from build123d import *

# Parameters (mm, degrees)
PAD_DEPTH       = 12
POCKET_DEPTH    = 10.1
POCKET001_DEPTH = 10.1
SKETCH003_W     = 15.841853
SKETCH003_H     = 14.91592
POCKET002_DEPTH = 4
SKETCH004_R     = 2
PAD001_DEPTH    = 2
CHAMFER_SIZE    = 0.5
CHAMFER001_SIZE = 1


with BuildPart() as part:
    # Sketch → Pad (new body)
    with BuildSketch(Plane.XY):
        Polygon((0, 7), (10, 7), (10, 0), (0, -10), (-7, -10), (-7, 0), (-4, 0), (0, 4), align=None)
    extrude(amount=PAD_DEPTH)

    # Sketch001 (on Face4 of Pad) → Pocket (cut)
    with BuildSketch(Plane.XZ.offset(10)):
        with BuildLine():
            Line((-4.5, 10), (-4.5, 13.32))
            Line((-4.5, 13.32), (-4, 13.32))
            Line((-4, 13.32), (-4, 4))
            ThreePointArc((-5, 4), (-4.5, 3.5), (-4, 4))
            Line((-5, 4), (-5, 9.5))
            Line((-5, 9.5), (-4.5, 10))
        make_face()
    extrude(amount=-POCKET_DEPTH, mode=Mode.SUBTRACT)

    # Sketch002 (on Face3 of Pocket) → Pocket001 (cut)
    with BuildSketch(Plane.YZ.offset(10)):
        with BuildLine():
            Line((4.5, 12.95), (4.5, 10))
            Line((4.5, 10), (5, 9.5))
            Line((5, 9.5), (5, 4))
            ThreePointArc((4, 4), (4.5, 3.5), (5, 4))
            Line((4, 4), (4, 12.95))
            Line((4, 12.95), (4.5, 12.95))
        make_face()
    extrude(amount=-POCKET001_DEPTH, mode=Mode.SUBTRACT)

    # Sketch003 (on Face5 of Pocket001) → Pocket002 (cut)
    with BuildSketch(Plane.XY.offset(12)):
        with Locations((3.700034, -3.226885)):
            Rectangle(SKETCH003_W, SKETCH003_H)
    extrude(amount=-POCKET002_DEPTH, mode=Mode.SUBTRACT)

    # Sketch004 (on Face12 of Pocket002) → Pad001 (join)
    with BuildSketch(Plane.XY.offset(8)):
        Circle(SKETCH004_R)
    extrude(amount=PAD001_DEPTH)

    # Chamfer
    chamfer_edges = [part.edges().sort_by_distance(p)[0] for p in [
        (-2, 0, 10),
    ]]
    chamfer(chamfer_edges, length=CHAMFER_SIZE)

    # Chamfer001
    chamfer001_edges = [part.edges().sort_by_distance(p)[0] for p in [
        (-7, -10, 6),
        (-7, 0, 6),
        (0, 7, 6),
        (10, 7, 6),
        (5, 4.5, 12),
        (-4.5, -5, 12),
    ]]
    chamfer(chamfer001_edges, length=CHAMFER001_SIZE)


solid = part.part
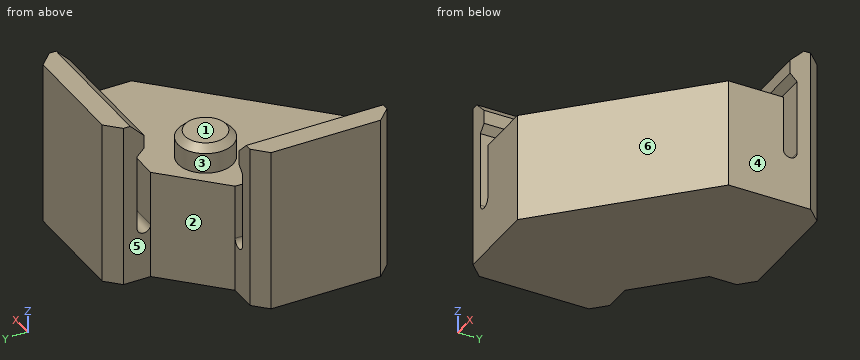
Design review of the part built by this model. Coordinates are the model's own, in mm. Face numbers are marked on the shaded views. A direction names the side the tool comes from. Round coordinates to 2 decimals unless told otherwise and drop trailing zeros. Order: outer loops, then holes, each group sorted by start corner. A loop starts at its lowest first (then second) coordinate and runs counter-clockwise, first axis right, second up.
1) Consider section D-D (z = 1.25). State the section outline as (x, y) points, plus the area to 3 significant figures.
The answers:
outline: (-7, -9) - (-6, -10) - (0, -10) - (10, 0) - (10, 6) - (9, 7) - (1, 7) - (0, 6) - (0, 4) - (-4, 0) - (-6, 0) - (-7, -1) - close
area: 196 mm2
2) Clearance check with flat-ended pins moving along their axes: pin 1 Ø1.6 at (y, z) = (5, 7) entering from -X; pin 2 Ø4 at (y, z) = (-7, 8.5) entering from +X; pin 3 Ø6 at (x, z) = (4, 7.5) entering from -Y. State where each tip first meets the part, or that it passes through.
The answers:
pin 1: stops at x = 0
pin 2: stops at x = 4.94
pin 3: stops at y = -9
3) For L1, parallel to Y at x = -5.5, z = 4; L2, parallel to Z at x = 6, y = -2.75; L3, parallel to Y at x = -3, z = 2, list the stretches that pass through material, from the lowest coordinate up.
The answers:
L1: y = -10 to 0
L2: z = 0 to 8
L3: y = -10 to 1
4) Consider section A-A (z = 6.75). State the section outline as (x, y) points.
The answers:
outline: (-7, -9) - (-6, -10) - (-5, -10) - (-5, 0) - (-6, 0) - (-7, -1) - close; (-4, -10) - (0, -10) - (10, 0) - (10, 4) - (0, 4) - (-4, 0) - close; (0, 5) - (10, 5) - (10, 6) - (9, 7) - (1, 7) - (0, 6) - close
5) Consider section C-C (x = -2.25). State the section outline as (y, z) points, plus the area to 3 significant figures.
The answers:
outline: (-10, 0) - (1.75, 0) - (1.75, 8) - (-10, 8) - close
area: 94.0 mm2
6) Consider section B-B (y = -3.25). State the section outline as (x, z) points, plus the area to 3 significant figures.
The answers:
outline: (-7, 0) - (6.75, 0) - (6.75, 8) - (-4, 8) - (-4, 4) arc R0.5 cw to (-5, 4) - (-5, 9.5) - (-4.5, 10) - (-4.5, 11) - (-5.5, 12) - (-7, 12) - close
area: 114 mm2
7) Draft analysis for pull direction X (two halves, no side actions). For the marked faces 1, 2, 3 and 4, state which applies: released by +X, released by -X, zero draft, split by the parting line, or undercut.
The answers:
face 1: zero draft
face 2: released by -X
face 3: undercut
face 4: released by +X
8) Machinability: for the marked faces 5 and 6, which of the approach directions +Z, -Z, +X, -X, +Y, -Y give a long, thin tool a straight path to every point of the face, cutting with its end or side? Answer none if there is none.
The answers:
face 5: +Z, -Z, -X, +Y
face 6: +Z, -Z, +X, -Y
